Design review of the part built by this model. Coordinates are the model's own, in mm. Round coordinates to 2 decimals unless told otherwise and drop trailing zeros. Loops run counter-clockwise (first coordinate to the right, second up) from the corner with the lowest first, then second, coordinate; pieces in that order, holes last. Notation, with made-up numbers: (12, 38) - (47, 38) arc R16 cw to (47, 57) - close; hole circle Ø9 at (85, 11.25). An arc over 180 degrees is marked (long way). Return JSON: item names as keys, results as strings. Group by question number.
from build123d import *

# Parameters (mm, degrees)
SKETCH1_W           = 19.05
SKETCH1_H           = 6.35
BOSS_EXTRUDE1_DEPTH = 3.175


with BuildPart() as part:
    # Sketch1 → Boss-Extrude1 (new, symmetric)
    with BuildSketch(Plane.XY):
        Rectangle(SKETCH1_W, SKETCH1_H)
    extrude(amount=BOSS_EXTRUDE1_DEPTH, both=True)


with BuildPart() as body_2:
    # Sketch2 → Revolve2 (revolve)
    with BuildSketch(Plane.XY, mode=Mode.PRIVATE) as revolve2_sk:
        with BuildLine():
            Line((-12.5, 0), (12.5, 0))
            ThreePointArc((12.5, 0), (11.035533906, 3.535533906), (7.5, 5))
            Line((7.5, 5), (-7.5, 5))
            ThreePointArc((-7.5, 5), (-11.035533906, 3.535533906), (-12.5, 0))
        make_face()
    revolve(revolve2_sk.sketch.rotate(Axis((-12.5, 0, 0), (1, 0, 0)), 180), axis=Axis((-12.5, 0, 0), (1, 0, 0)))

    # Combine1: cut part
    add(part.part, mode=Mode.SUBTRACT)


solid = body_2.part
Q1. For line 1 (X direction, y = 1.5, z = -2.25) (3 decimals); line 2 (Z direction, x = 0.5, y = 1.25) (3 decimals); line 3 (Y direction, x = -7, z = 1) (3 decimals), list the stretches that pass through material, from the lowest coordinate up.
Q2. Draft analysis for pull direction X (two halves, no side actions). For faces 1 (the cylindrical face through (0, 5, 0)), 2 (the flat face through (9.525, 0, 0)), state which applies: pulls with the +X half, pulls with the -X half, needs draft (parallel to the pull), parting line crosses it, or undercut.
Q3. Insertion check: pin 1 Ø2 at (x, z) = (-4, -3) entering from -Y; pin 2 Ø3 at (x, y) = (6.5, 2.5) entering from +Z; pin 3 Ø1.5 at (x, z) = (4, 3.5) entering from -Y. Each pin has a flat end and moves straight along its axis. Give the tip position at first contact, or say it passes through.
Q4. Add section B-B, the plane x = -4. State the section outline as (y, z) points (3 decimals), plus the area to 3 significant figures.
Q5. Add section D-D, the plane y = 1.75. State the section outline as (x, z) points (1 decimal).
Evaluation:
{
 "1": {"line 1": "-11.706 to -9.525, 9.525 to 11.706", "line 2": "-4.841 to -3.175, 3.175 to 4.841", "line 3": "-4.899 to -3.175, 3.175 to 4.899"},
 "2": {"face 1": "needs draft", "face 2": "undercut"},
 "3": {"pin 1": "y = -4.58", "pin 2": "z = 4.9", "pin 3": "y = -4.18"},
 "4": {"outline": "circle Ø10 at (0, 0); hole (-3.175, -3.175) - (3.175, -3.175) - (3.175, 3.175) - (-3.175, 3.175) - close", "area": "38.2 mm²"},
 "5": {"outline": "(-7.5, -4.7) - (7.5, -4.7) arc R4.7 ccw to (7.5, 4.7) - (-7.5, 4.7) arc R4.7 ccw to start; hole (-9.5, -3.2) - (9.5, -3.2) - (9.5, 3.2) - (-9.5, 3.2) - close"}
}
